from build123d import *

# Parameters (mm, degrees)
BOSS_EXTRUDE1_DEPTH = 180
FILLET1_R           = 0.3


with BuildPart() as part:
    # Sketch1 → Boss-Extrude1 (new body)
    with BuildSketch(Plane.XY):
        Polygon((-8.3, 1), (8.3, 1), (8.3, 0), (7, 0), (7, -1.3), (7.5, -1.8), (6.883716857, -4.1), (6, -4.1), (6, 0), (-6, 0), (-6, -4.1), (-6.883716857, -4.1), (-7.5, -1.8), (-7, -1.3), (-7, 0), (-8.3, 0), align=None)
    extrude(amount=BOSS_EXTRUDE1_DEPTH)

    # Fillet1
    fillet1_edges = [part.edges().sort_by_distance(p)[0] for p in [
        (-8.3, 1, 90),
        (8.3, 1, 90),
        (7, -1.3, 90),
        (7.5, -1.8, 90),
        (6.883716857, -4.1, 90),
        (6, -4.1, 90),
        (6, 0, 90),
        (-6, 0, 90),
        (-6, -4.1, 90),
        (-6.883716857, -4.1, 90),
        (-7.5, -1.8, 90),
        (-7, -1.3, 90),
    ]]
    fillet(fillet1_edges, radius=FILLET1_R)


solid = part.part
For this review, take the finished solid that the model builds, in its own axes (mm). A direction names the side the tool comes from. Round coordinates to 2 decimals unless told otherwise and drop trailing zeros. Write each loop counter-clockwise with the first axis right and the second up, starting at its lowest first coordinate (ties: lowest second). Pieces come first, ordered by that corner, then holes. Notation, with made-up numbers: M 88.25,-8.5 L 132.25,-8.5 A10 cw 132.25,0.5 Z; hole C 22.5,48.25 d5. An arc over 180 degrees is marked long. Write item = value, one per line. Start each with the question number.
(1) For faces 3 (the face through (0, 0.4, 180)), 4 (the face through (6, -2, 89)), list the 3-axis set-ups (+Z, -Z, +X, -X, +Y, -Y) from which the entire face can be reached by the end or side of a thin tool; tool diameter is ignored.
(2) We need section B-B (x = 0.75). Give the boundary of the cut face in (y, z).
(3) Clearance check with flat-ended pins moving along their axes: pin 1 Ø0.6 at (y, z) = (-0.5, 52) entering from +X; pin 2 Ø1.3 at (y, z) = (-1, 101) entering from -X; pin 3 Ø1 at (y, z) = (-2.5, 30) entering from +X; pin 4 Ø2 at (x, y) = (-3.5, 0) entering from -Z. State where each tip first meets the part, or that it passes through.
(4) The part is to be moulded in two halves that separate along X. For faces 1 (the face through (0, 1, 89)), 2 (the face through (-6, -2, 89)), say which applies: +X half, -X half, draft (parallel to the pull), parting line (faces both ways), or undercut.
(5) We need section A-A (z = 144). Give the boundary of the cut face in (x, y).
(6) For line 1 along X through (y, z) = (-1.3, 83.5); line 2 along Y through (x, z) = (-5.75, 60.5); line 3 along X through (y, z) = (-2.65, 119), list the stretches that pass through material, from the lowest coordinate up.
Results found:
q1.face_3 = +Z, +X, -X, +Y, -Y
q1.face_4 = +Z, -Z, -Y
q2.outline = M 0,0 L 1,0 L 1,180 L 0,180 Z
q3.pin_1 = 7
q3.pin_2 = -7.35
q3.pin_3 = 7.45
q3.pin_4 = 0
q4.face_1 = draft
q4.face_2 = undercut
q5.outline = M -8.3,0 L -7,0 L -7,-1.18 A0.3 cw -7.09,-1.39 L -7.38,-1.68 A0.3 ccw -7.46,-1.97 L -6.94,-3.88 A0.3 ccw -6.65,-4.1 L -6.3,-4.1 A0.3 ccw -6,-3.8 L -6,-0.3 A0.3 cw -5.7,0 L 5.7,0 A0.3 cw 6,-0.3 L 6,-3.8 A0.3 ccw 6.3,-4.1 L 6.65,-4.1 A0.3 ccw 6.94,-3.88 L 7.46,-1.97 A0.3 ccw 7.38,-1.68 L 7.09,-1.39 A0.3 cw 7,-1.18 L 7,0 L 8.3,0 L 8.3,0.7 A0.3 ccw 8,1 L -8,1 A0.3 ccw -8.3,0.7 Z
q6.line_1 = -7.03 to -6, 6 to 7.03
q6.line_2 = 0 to 1
q6.line_3 = -7.27 to -6, 6 to 7.27
